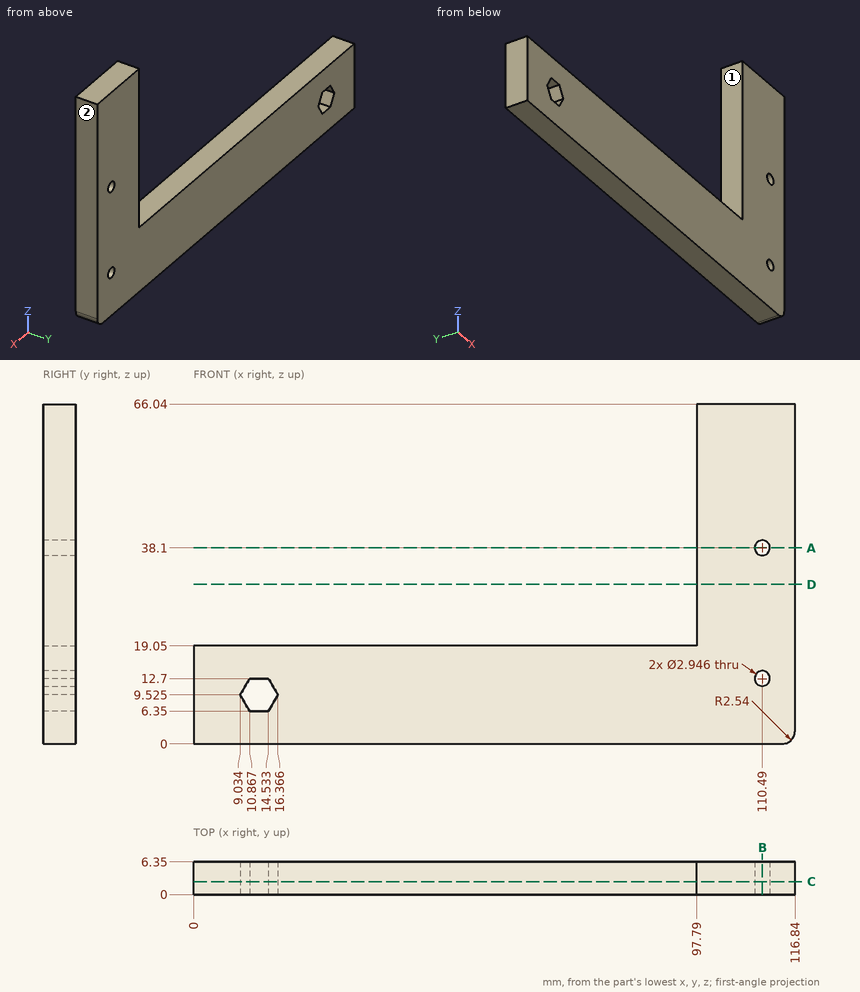
Study the drawing (mm; zero at the part's minimum x, y, z) and answer. A direction names the side the tool comes from. Give positions to 0.01 mm unless a question says otherwise; leave off trailing zeros. Order: outer loops, then holes, each group sorted by start corner. A loop starts at its lowest first (then second) coordinate and runs counter-clockwise, first axis right, second up. Notation, with made-up numbers: M 89,31.5 L 124,31.5 A20 ccw 124,62.5 Z; hole C 68.25,-7 d5. An arc over 180 degrees is marked long. Put each result on its own line as item: value. Start each with the question number.
Item 1: Which of the six approach directions +Z, -Z, +X, -X, +Y, -Y give full straight-line access (tool end or side, diameter ignored) to the marked faces 1 and 2?
Item 2: The part is cut by section B-B, the plane x = 110.49. Determine the outline of the cut face in (y, z), and give its area (3 significant figures).
Item 3: Find the intervals of material crossed by line 1 along Z through (x, y) = (110.49, 4.5); line 2 along X through (y, z) = (3.75, 38.1); line 3 along Z through (x, y) = (57, 3), in increasing order.
Item 4: The part is cut by section A-A, the plane z = 38.1. Determine the outline of the cut face in (x, y), and give its area (3 significant figures).
Item 5: Flat-ended cylindrical pins translate along their axes: P1, Ø2.5, axis at x = 110.49, z = 12.7, coming from the +Y side; P2, Ø1.5, axis at x = 59.5, y = 5, coming from the +Z side; P3, Ø3, axis at y = 4.5, z = 38.5, coming from the -X side. Find the tip coordinate at first contact, or state that the pin passes through.
Item 6: The part is cut by section C-C, the plane y = 2.5. State how many separate pieces and enclosed holes the cut face has, and give its area (3 significant figures).
Item 7: The part is cut by section D-D, the plane z = 31. Determine the outline of the cut face in (x, y).
Answer key:
1. face 1: +Z, -X, +Y, -Y
1. face 2: +Z, -Z, +X, +Y, -Y
2. outline: M 0,0 L 6.35,0 L 6.35,11.23 L 0,11.23 Z; M 0,14.17 L 6.35,14.17 L 6.35,36.63 L 0,36.63 Z; M 0,39.57 L 6.35,39.57 L 6.35,66.04 L 0,66.04 Z
2. area: 382 mm²
3. line 1: z = 0 to 11.23, 14.17 to 36.63, 39.57 to 66.04
3. line 2: x = 97.79 to 109.02, 111.96 to 116.84
3. line 3: z = 0 to 19.05
4. outline: M 97.79,0 L 109.02,0 L 109.02,6.35 L 97.79,6.35 Z; M 111.96,0 L 116.84,0 L 116.84,6.35 L 111.96,6.35 Z
4. area: 102 mm²
5. P1: passes through
5. P2: stops at z = 19.05
5. P3: stops at x = 97.79
6. separate pieces: 1
6. enclosed holes: 3
6. area: 3,070 mm²
7. outline: M 97.79,0 L 116.84,0 L 116.84,6.35 L 97.79,6.35 Z
